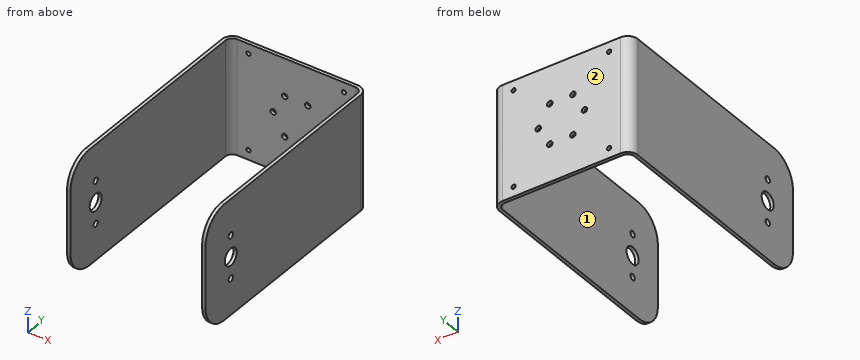
from build123d import *

# Parameters (mm, degrees)
SKETCH3_W                    = 130
SKETCH3_H                    = 107.95
BASE_FLANGE1_DEPTH           = 3.175
EDGE_FLANGE1_STRIP_W         = 25.4
EDGE_FLANGE1_STRIP_H         = 3.175
EDGE_FLANGE1_STRIP_CUT_DEPTH = 107.95
EDGE_FLANGE1_DEPTH           = 107.95
EDGE_FLANGE1_PROFILE_W       = 107.95
EDGE_FLANGE1_PROFILE_H       = 204.7875
EDGE_FLANGE1_PROFILE_R       = 2.855235605
EDGE_FLANGE1_PROFILE_R_2     = 7.9375
EDGE_FLANGE1_FLAT_DEPTH      = 3.175
FILLET1_R                    = 25
SKETCH13_R                   = 2.6
FLANGE_COUPLING_HOLES_DEPTH  = 231.365249726
SKETCH15_R                   = 1.985
CUT_EXTRUDE1_DEPTH           = 231.365249726


# Sheet-metal steps are written as plain solids
with BuildPart() as part:
    # Sketch3 → Base-Flange1 (new body)
    with BuildSketch(Plane(origin=(0, 0, 0), x_dir=(1, 0, 0), z_dir=(0, 1, 0))):
        Rectangle(SKETCH3_W, SKETCH3_H)
    extrude(amount=-BASE_FLANGE1_DEPTH)

    # Edge-Flange1 strip (across the edge) → Edge-Flange1 strip cut (cut)
    with BuildSketch(Plane(origin=(65, -3.175, -53.975), x_dir=(-1, 0, 0), z_dir=(0, 0, 1))):
        with Locations((-3.175, -1.5875)):
            Rectangle(EDGE_FLANGE1_STRIP_W, EDGE_FLANGE1_STRIP_H)
    edge_flange1_strip_cut = extrude(amount=EDGE_FLANGE1_STRIP_CUT_DEPTH, mode=Mode.SUBTRACT)

    # Edge-Flange1 bend section (across the edge) → Edge-Flange1 (add)
    with BuildSketch(Plane(origin=(65, -3.175, -53.975), x_dir=(-1, 0, 0), z_dir=(0, 0, 1))):
        with BuildLine():
            Line((0, 6.35), (3.175, 6.35))
            ThreePointArc((3.175, 6.35), (5.034871939, 1.859871939), (9.525, 0))
            Line((9.525, 0), (9.525, -3.175))
            ThreePointArc((9.525, -3.175), (2.789807909, -0.385192091), (0, 6.35))
        make_face()
    edge_flange1 = extrude(amount=EDGE_FLANGE1_DEPTH)

    # Edge-Flange1 profile (on flange) → Edge-Flange1 flat (add)
    with BuildSketch(Plane(origin=(65, -3.175, 0), x_dir=(0, 0, -1), z_dir=(-1, 0, 0))):
        with Locations((0, 108.74375)):
            Rectangle(EDGE_FLANGE1_PROFILE_W, EDGE_FLANGE1_PROFILE_H)
        with Locations((20, 177.8)):
            Circle(EDGE_FLANGE1_PROFILE_R, mode=Mode.SUBTRACT)
        with Locations((0, 177.8)):
            Circle(EDGE_FLANGE1_PROFILE_R_2, mode=Mode.SUBTRACT)
        with Locations((-20, 177.8)):
            Circle(EDGE_FLANGE1_PROFILE_R, mode=Mode.SUBTRACT)
    edge_flange1_flat = extrude(amount=EDGE_FLANGE1_FLAT_DEPTH)

    # Mirror1: Edge-Flange1 strip cut, Edge-Flange1, Edge-Flange1 flat across plane
    add(edge_flange1_strip_cut.mirror(Plane(origin=(0, 0, 0), x_dir=(0, 0, 1), z_dir=(1, 0, 0))), mode=Mode.SUBTRACT)
    add(edge_flange1.mirror(Plane(origin=(0, 0, 0), x_dir=(0, 0, 1), z_dir=(1, 0, 0))))
    add(edge_flange1_flat.mirror(Plane(origin=(0, 0, 0), x_dir=(0, 0, 1), z_dir=(1, 0, 0))))

    # Fillet1
    fillet1_edges = [part.edges().sort_by_distance(p)[0] for p in [
        (-63.4125, -214.3125, -53.975),
        (63.4125, -214.3125, -53.975),
        (63.4125, -214.3125, 53.975),
        (-63.4125, -214.3125, 53.975),
    ]]
    fillet(fillet1_edges, radius=FILLET1_R)

    # Sketch13 → Flange Coupling Holes (cut, through all)
    with BuildSketch(Plane(origin=(0, 0, 0), x_dir=(1, 0, 0), z_dir=(0, 1, 0))):
        with Locations(Location((-21.7, 0, 0), (0, 0, 270))):
            Circle(SKETCH13_R)
        with Locations(Location((-10.85, 18.792751262, 0), (0, 0, 270))):
            Circle(SKETCH13_R)
        with Locations(Location((10.85, 18.792751262, 0), (0, 0, 270))):
            Circle(SKETCH13_R)
        with Locations(Location((21.7, 0, 0), (0, 0, 270))):
            Circle(SKETCH13_R)
        with Locations(Location((10.85, -18.792751262, 0), (0, 0, 270))):
            Circle(SKETCH13_R)
        with Locations(Location((-10.85, -18.792751262, 0), (0, 0, 270))):
            Circle(SKETCH13_R)
    extrude(amount=-FLANGE_COUPLING_HOLES_DEPTH, mode=Mode.SUBTRACT)

    # Sketch15 → Cut-Extrude1 (cut, through all)
    with BuildSketch(Plane(origin=(0, 0, 0), x_dir=(1, 0, 0), z_dir=(0, 1, 0))):
        with Locations(Location((-44.845, 44.845, 0), (0, 0, 270))):
            Circle(SKETCH15_R)
        with Locations(Location((44.845, 44.845, 0), (0, 0, 270))):
            Circle(SKETCH15_R)
        with Locations(Location((44.845, -44.845, 0), (0, 0, 270))):
            Circle(SKETCH15_R)
        with Locations(Location((-44.845, -44.845, 0), (0, 0, 270))):
            Circle(SKETCH15_R)
    extrude(amount=-CUT_EXTRUDE1_DEPTH, mode=Mode.SUBTRACT)


solid = part.part
Can you work these out from the model? Positions are in its coordinate system, mm. Face numbers are marked on the shaded views. A direction names the side the tool comes from. Give positions to 0.01 mm unless a question says otherwise; leave off trailing zeros. Write each loop counter-clockwise with the first axis right and the second up, starting at its lowest first coordinate (ties: lowest second). Pieces come first, ordered by that corner, then holes. Notation, with made-up numbers: (88.5, 15) -> (101.5, 15) arc R19 ccw to (101.5, 31) -> close; hole circle Ø11 at (-22, -35). An arc over 180 degrees is marked (long way). Answer as a JSON object with one key per item and string values. Group by question number.
Item 1: Please list where these lines run through material, in increasing order: line 1 (X direction, y = -104, z = 30) (3 decimals); line 2 (Y direction, x = -38.5, z = -40) (3 decimals). Write a range as [from, to].
Item 2: Suppose I cut it at A-A (x = -21.7). Please give me the cut outline in (y, z) (3 decimals).
Item 3: Suppose I cut it at D-D (z = -33.5). Please give me the cut outline in (x, y) (3 decimals).
Item 4: I'm going to push flat-ended pins straight in: P1, Ø6, axis at x = -31.5, z = -4, coming from the -Y side (3 decimals); P2, Ø5, axis at y = -180.975, z = -20, coming from the +X side. Where does each tip first touch, or does it pass through?
Item 5: Suppose I cut it at C-C (y = -17). Please give me the cut outline in (x, z) (3 decimals), plus the area to 3 significant figures.
Item 6: Suppose I cut it at B-B (z = 0). State how many separate pieces and enclosed holes the cut face has, plus the area to 3 significant figures.
Item 7: For the marked faces 1 and 2, which set-ups out of +Z, -Z, +X, -X, +Y, -Y let a thin tool reach every point of the face, with its end or its side?
Findings:
{
 "1": {"line 1": "x = [-65, -61.825], [61.825, 65]", "line 2": "y = [-3.175, 0]"},
 "2": {"outline": "(-3.175, -53.975) -> (0, -53.975) -> (0, -2.6) -> (-3.175, -2.6) -> close; (-3.175, 2.6) -> (0, 2.6) -> (0, 53.975) -> (-3.175, 53.975) -> close"},
 "3": {"outline": "(-65, -213.9) -> (-61.825, -213.9) -> (-61.825, -9.525) arc R6.35 cw to (-55.475, -3.175) -> (55.475, -3.175) arc R6.35 cw to (61.825, -9.525) -> (61.825, -213.9) -> (65, -213.9) -> (65, -9.525) arc R9.525 ccw to (55.475, 0) -> (-55.475, 0) arc R9.525 ccw to (-65, -9.525) -> close"},
 "4": {"P1": "stops at y = -3.175", "P2": "passes through"},
 "5": {"outline": "(-65, -53.975) -> (-61.825, -53.975) -> (-61.825, 53.975) -> (-65, 53.975) -> close; (61.825, -53.975) -> (65, -53.975) -> (65, 53.975) -> (61.825, 53.975) -> close", "area": "685 mm²"},
 "6": {"separate pieces": "5", "enclosed holes": "0", "area": "1,600 mm²"},
 "7": {"face 1": "+Z, -Z, -Y", "face 2": "+Z, -Z, +X, -X, +Y"}
}
